Work out the finished part from the listing and answer in its coordinate system (mm). Face numbers are marked on the shaded views. A direction names the side the tool comes from. Give positions to 0.01 mm unless a question says otherwise; leave off trailing zeros. Loops run counter-clockwise (first coordinate to the right, second up) from the corner with the lowest first, then second, coordinate; pieces in that order, holes last. Notation, with made-up numbers: M 35,6 L 82,6 A10 ccw 82,21 Z; hole C -21.5,21 d7. An arc over 180 degrees is marked long. Use a Markdown table: item, result.
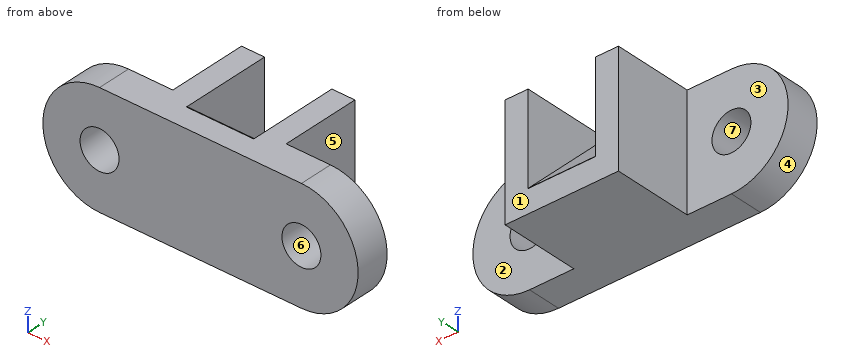
```python
from build123d import *

# Parameters (mm, degrees)
BOSS_EXTRUDE2_DEPTH = 19
SKETCH4_R           = 11
CUT_EXTRUDE1_DEPTH  = 151.668510313
SKETCH5_W           = 64
SKETCH5_H           = 64
BOSS_EXTRUDE3_DEPTH = 45
SKETCH6_W           = 38
SKETCH6_H           = 51
CUT_EXTRUDE2_DEPTH  = 51
BOSS_EXTRUDE4_DEPTH = 38


with BuildPart() as part:
    # Sketch3 → Boss-Extrude2 (new body)
    with BuildSketch(Plane(origin=(0, 0, 0), x_dir=(1, 0, 0), z_dir=(0, 1, 0))):
        with BuildLine():
            Line((0, 32), (114, 32))
            ThreePointArc((114, 32), (146, 0), (114, -32))
            Line((114, -32), (0, -32))
            ThreePointArc((0, -32), (-32, 0), (0, 32))
        make_face()
    extrude(amount=BOSS_EXTRUDE2_DEPTH)

    # Sketch4 → Cut-Extrude1 (cut, through all)
    with BuildSketch(Plane(origin=(0, 19, 0), x_dir=(1, 0, 0), z_dir=(0, 1, 0))):
        with Locations(Location((0, 0, 0), (0, 0, 270))):
            Circle(SKETCH4_R)
        with Locations(Location((114, 0, 0), (0, 0, 90))):
            Circle(SKETCH4_R)
    extrude(amount=-CUT_EXTRUDE1_DEPTH, mode=Mode.SUBTRACT)

    # Sketch5 → Boss-Extrude3 (add)
    with BuildSketch(Plane(origin=(0, 19, 0), x_dir=(1, 0, 0), z_dir=(0, 1, 0))):
        with Locations((57, 0)):
            Rectangle(SKETCH5_W, SKETCH5_H)
    extrude(amount=BOSS_EXTRUDE3_DEPTH)

    # Sketch6 → Cut-Extrude2 (cut)
    with BuildSketch(Plane.XY.offset(32)):
        with Locations((57, 38.5)):
            Rectangle(SKETCH6_W, SKETCH6_H)
    extrude(amount=-CUT_EXTRUDE2_DEPTH, mode=Mode.SUBTRACT)

    # Sketch8 → Boss-Extrude4 (add)
    with BuildSketch(Plane(origin=(38, 0, 0), x_dir=(0, 0, -1), z_dir=(1, 0, 0))):
        Polygon((18.549537032, 63.66671572), (-32.32969233, 12.787486357), (18.549537032, 15.77285286), align=None)
    extrude(amount=BOSS_EXTRUDE4_DEPTH)


solid = part.part
```
(1) A cutting plane is placed at B-B (y = 29). Write down the section's boundary in (x, z), and give its area (3 significant figures).
Entries:
| item | result |
|---|---|
| outline | M 25,-32 L 89,-32 L 89,32 L 76,32 L 76,16.12 L 38,16.12 L 38,32 L 25,32 Z; hole M 38,-19 L 76,-19 L 76,-18.55 L 38,-18.55 Z |
| area | 3,480 mm² |
(2) A cutting plane is placed at A-A (z = 0). Write down the section's boundary in (x, y).
Entries:
| item | result |
|---|---|
| outline | M -32,0 L -11,0 L -11,19 L -32,19 Z; M 11,0 L 103,0 L 103,19 L 89,19 L 89,64 L 76,64 L 76,45.12 L 38,45.12 L 38,64 L 25,64 L 25,19 L 11,19 Z; M 125,0 L 146,0 L 146,19 L 125,19 Z; hole M 38,13 L 76,13 L 76,14.68 L 38,14.68 Z |
(3) Consider probe 1 along X at (y, z) = (5, 0); probe 2 along Z at (x, y) = (114, 10.25); probe 3 along X at (y, z) = (30.5, -6.5). Determine where each line is inside the solid, lowest interval first. Write a range as [from, to].
Entries:
| item | result |
|---|---|
| probe 1 | x = [-32, -11], [11, 103], [125, 146] |
| probe 2 | z = [-32, -11], [11, 32] |
| probe 3 | x = [25, 89] |
(4) The mould has two halves that part along Z. Classify the marked faces 4, 5, 6 and 7: released by +Z, released by -Z, zero draft, split by the parting line, or undercut.
Entries:
| item | result |
|---|---|
| face 4 | split by the parting line |
| face 5 | zero draft |
| face 6 | undercut |
| face 7 | undercut |
(5) Given P1, Ø10, axis at y = 50, z = -9, coming from the -X side; P2, Ø17, axis at x = -3, z = 0, coming from the +Y side; P3, Ø10, axis at x = 65, y = 28, coming from the +Z side; P4, Ø2, axis at x = 35, z = 24, coming from the -Y side, each flat-ended and moving along its own axis, determine where each tip first touches the part or whether it passes through.
Entries:
| item | result |
|---|---|
| P1 | stops at x = 25 |
| P2 | stops at y = 19 |
| P3 | stops at z = 22.12 |
| P4 | stops at y = 0 |
(6) A cutting plane is placed at D-D (z = 16.5). Write down the section's boundary in (x, y), and give its area (3 significant figures).
Entries:
| item | result |
|---|---|
| outline | M -27.42,0 L 141.42,0 L 141.42,19 L 89,19 L 89,64 L 76,64 L 76,28.62 L 38,28.62 L 38,64 L 25,64 L 25,19 L -27.42,19 Z; hole M 38,13 L 76,13 L 76,13.72 L 38,13.72 Z |
| area | 4,720 mm² |
(7) A cutting plane is placed at C-C (x = 40). Write down the section's boundary in (y, z), and give its area (3 significant figures).
Entries:
| item | result |
|---|---|
| outline | M 0,-32 L 64,-32 L 64,-19 L 13,-19 L 13,28.71 L 15.77,-18.55 L 63.67,-18.55 L 12.79,32.33 L 12.81,32 L 0,32 Z |
| area | 2,710 mm² |
(8) Which of the six approach directions +Z, -Z, +X, -X, +Y, -Y give full straight-line access (tool end or side, diameter ignored) to the marked faces 1, 2 and 3?
Entries:
| item | result |
|---|---|
| face 1 | +Z, -Z, +X, -X, +Y |
| face 2 | +Z, -Z, +X, +Y |
| face 3 | +Z, -Z, -X, +Y |
